CAD build for the part. Positions are in the model's coordinates, mm. Face numbers are marked on the shaded views. A direction names the side the tool comes from. Give positions to 0.01 mm unless a question says otherwise; leave off trailing zeros. Order: outer loops, then holes, each group sorted by start corner. A loop starts at its lowest first (then second) coordinate and runs counter-clockwise, first axis right, second up. Notation, with made-up numbers: M 41,-14 L 60,-14 A35 ccw 60,24 Z; hole C 66.5,87.25 d3. An arc over 180 degrees is marked long. Put each result on its own line as item: value. Start each with the question number.
1) Cut at B-B (y = 13.5). Give the number of separate pieces and of enclosed holes in the cut face, and give its area (3 significant figures).
2) Cut at C-C (z = 2.75). Write the cut outline in (x, y).
3) Pin check, flat tips, straight feed: pin 1 (5 mm diameter, centred on x = 19.5, z = -4, fed in from -Y); pin 2 (3.5 mm diameter, centred on x = -24.5, z = 0, fed in from +Y); pin 3 (1.5 mm diameter, centred on y = 4, z = -3.5, fed in from +X). Stop position of each tip, or through.
4) Cut at A-A (x = -16.5). Write the cut outline in (y, z), and give its area (3 significant figures).
5) Drill centre lines: line 1 (Z direction, x = -19.5, y = 13); line 2 (Y direction, x = 6.5, z = -1); line 3 (X direction, y = 3.5, z = -2.25). Where is each one in solid material? Low to high. Write a range as [from, to].
6) Tool access for the marked faces 1 and 2: list every direction of +Z, -Z, +X, -X, +Y, -Y with a clear straight run to the whole face (end or side of a thin tool).
7) Cut at D-D (x = 8.5). Write the cut outline in (y, z).
```python
from build123d import *

# Parameters (mm, degrees)
SKETCH2_R           = 5
BOSS_EXTRUDE1_DEPTH = 8.44
SKETCH3_R           = 5
BOSS_EXTRUDE2_DEPTH = 6
BOSS_EXTRUDE3_DEPTH = 3
CUT_EXTRUDE1_REACH  = 35.805
SKETCH5_R           = 1.5
SKETCH6_R           = 5
BOSS_EXTRUDE4_DEPTH = 1


with BuildPart() as part:
    # Sketch2 → Boss-Extrude1 (new body)
    with BuildSketch(Plane(origin=(0, 0, 0), x_dir=(1, 0, 0), z_dir=(0, 1, 0))):
        with Locations(Location((0, 0, 0), (0, 0, 270))):
            Circle(SKETCH2_R)
    extrude(amount=BOSS_EXTRUDE1_DEPTH)

    # Sketch3 → Boss-Extrude2 (add)
    with BuildSketch(Plane(origin=(0, 8.44, 0), x_dir=(1, 0, 0), z_dir=(0, 1, 0))):
        with Locations(Location((0, 0, 0), (0, 0, 270))):
            Circle(SKETCH3_R)
    extrude(amount=BOSS_EXTRUDE2_DEPTH)

    # Sketch4 → Boss-Extrude3 (add)
    with BuildSketch(Plane(origin=(0, 14.44, 0), x_dir=(1, 0, 0), z_dir=(0, 1, 0))):
        with BuildLine():
            Line((-0.979591837, -7.939798476), (-25.112244898, -4.962374047))
            ThreePointArc((-25.112244898, -4.962374047), (-29.5, 0), (-25.112244898, 4.962374047))
            Line((-25.112244898, 4.962374047), (-0.979591837, 7.939798476))
            ThreePointArc((-0.979591837, 7.939798476), (0, 8), (0.979591837, 7.939798476))
            Line((0.979591837, 7.939798476), (25.112244898, 4.962374047))
            ThreePointArc((25.112244898, 4.962374047), (29.5, 0), (25.112244898, -4.962374047))
            Line((25.112244898, -4.962374047), (0.979591837, -7.939798476))
            ThreePointArc((0.979591837, -7.939798476), (0, -8), (-0.979591837, -7.939798476))
        make_face()
    extrude(amount=-BOSS_EXTRUDE3_DEPTH)

    # Sketch5 → Cut-Extrude1 (cut, up to next)
    with BuildSketch(Plane(origin=(0, 14.44, 0), x_dir=(1, 0, 0), z_dir=(0, 1, 0)), mode=Mode.PRIVATE) as cut_extrude1_sk1:
        with Locations(Location((24.5, 0, 0), (0, 0, 270))):
            Circle(SKETCH5_R)
    cut_extrude1_tool1 = extrude(cut_extrude1_sk1.sketch, amount=-CUT_EXTRUDE1_REACH, mode=Mode.PRIVATE) & part.part
    # Sketch5 → Cut-Extrude1 (cut, up to next)
    with BuildSketch(Plane(origin=(0, 14.44, 0), x_dir=(1, 0, 0), z_dir=(0, 1, 0)), mode=Mode.PRIVATE) as cut_extrude1_sk2:
        with Locations(Location((20.5, 0, 0), (0, 0, 270))):
            Circle(SKETCH5_R)
    cut_extrude1_tool2 = extrude(cut_extrude1_sk2.sketch, amount=-CUT_EXTRUDE1_REACH, mode=Mode.PRIVATE) & part.part
    # Sketch5 → Cut-Extrude1 (cut, up to next)
    with BuildSketch(Plane(origin=(0, 14.44, 0), x_dir=(1, 0, 0), z_dir=(0, 1, 0)), mode=Mode.PRIVATE) as cut_extrude1_sk3:
        with Locations(Location((16.5, 0, 0), (0, 0, 270))):
            Circle(SKETCH5_R)
    cut_extrude1_tool3 = extrude(cut_extrude1_sk3.sketch, amount=-CUT_EXTRUDE1_REACH, mode=Mode.PRIVATE) & part.part
    # Sketch5 → Cut-Extrude1 (cut, up to next)
    with BuildSketch(Plane(origin=(0, 14.44, 0), x_dir=(1, 0, 0), z_dir=(0, 1, 0)), mode=Mode.PRIVATE) as cut_extrude1_sk4:
        with Locations(Location((12.5, 0, 0), (0, 0, 270))):
            Circle(SKETCH5_R)
    cut_extrude1_tool4 = extrude(cut_extrude1_sk4.sketch, amount=-CUT_EXTRUDE1_REACH, mode=Mode.PRIVATE) & part.part
    # Sketch5 → Cut-Extrude1 (cut, up to next)
    with BuildSketch(Plane(origin=(0, 14.44, 0), x_dir=(1, 0, 0), z_dir=(0, 1, 0)), mode=Mode.PRIVATE) as cut_extrude1_sk5:
        with Locations(Location((8.5, 0, 0), (0, 0, 270))):
            Circle(SKETCH5_R)
    cut_extrude1_tool5 = extrude(cut_extrude1_sk5.sketch, amount=-CUT_EXTRUDE1_REACH, mode=Mode.PRIVATE) & part.part
    # Sketch5 → Cut-Extrude1 (cut, up to next)
    with BuildSketch(Plane(origin=(0, 14.44, 0), x_dir=(1, 0, 0), z_dir=(0, 1, 0)), mode=Mode.PRIVATE) as cut_extrude1_sk6:
        with Locations(Location((-24.5, 0, 0), (0, 0, 270))):
            Circle(SKETCH5_R)
    cut_extrude1_tool6 = extrude(cut_extrude1_sk6.sketch, amount=-CUT_EXTRUDE1_REACH, mode=Mode.PRIVATE) & part.part
    # Sketch5 → Cut-Extrude1 (cut, up to next)
    with BuildSketch(Plane(origin=(0, 14.44, 0), x_dir=(1, 0, 0), z_dir=(0, 1, 0)), mode=Mode.PRIVATE) as cut_extrude1_sk7:
        with Locations(Location((-8.5, 0, 0), (0, 0, 270))):
            Circle(SKETCH5_R)
    cut_extrude1_tool7 = extrude(cut_extrude1_sk7.sketch, amount=-CUT_EXTRUDE1_REACH, mode=Mode.PRIVATE) & part.part
    # Sketch5 → Cut-Extrude1 (cut, up to next)
    with BuildSketch(Plane(origin=(0, 14.44, 0), x_dir=(1, 0, 0), z_dir=(0, 1, 0)), mode=Mode.PRIVATE) as cut_extrude1_sk8:
        with Locations(Location((-12.5, 0, 0), (0, 0, 270))):
            Circle(SKETCH5_R)
    cut_extrude1_tool8 = extrude(cut_extrude1_sk8.sketch, amount=-CUT_EXTRUDE1_REACH, mode=Mode.PRIVATE) & part.part
    # Sketch5 → Cut-Extrude1 (cut, up to next)
    with BuildSketch(Plane(origin=(0, 14.44, 0), x_dir=(1, 0, 0), z_dir=(0, 1, 0)), mode=Mode.PRIVATE) as cut_extrude1_sk9:
        with Locations(Location((-16.5, 0, 0), (0, 0, 270))):
            Circle(SKETCH5_R)
    cut_extrude1_tool9 = extrude(cut_extrude1_sk9.sketch, amount=-CUT_EXTRUDE1_REACH, mode=Mode.PRIVATE) & part.part
    # Sketch5 → Cut-Extrude1 (cut, up to next)
    with BuildSketch(Plane(origin=(0, 14.44, 0), x_dir=(1, 0, 0), z_dir=(0, 1, 0)), mode=Mode.PRIVATE) as cut_extrude1_sk10:
        with Locations(Location((-20.5, 0, 0), (0, 0, 270))):
            Circle(SKETCH5_R)
    cut_extrude1_tool10 = extrude(cut_extrude1_sk10.sketch, amount=-CUT_EXTRUDE1_REACH, mode=Mode.PRIVATE) & part.part
    add(cut_extrude1_tool1.solids().sort_by_distance((24.5, 14.44, 0))[0], mode=Mode.SUBTRACT)
    add(cut_extrude1_tool2.solids().sort_by_distance((20.5, 14.44, 0))[0], mode=Mode.SUBTRACT)
    add(cut_extrude1_tool3.solids().sort_by_distance((16.5, 14.44, 0))[0], mode=Mode.SUBTRACT)
    add(cut_extrude1_tool4.solids().sort_by_distance((12.5, 14.44, 0))[0], mode=Mode.SUBTRACT)
    add(cut_extrude1_tool5.solids().sort_by_distance((8.5, 14.44, 0))[0], mode=Mode.SUBTRACT)
    add(cut_extrude1_tool6.solids().sort_by_distance((-24.5, 14.44, 0))[0], mode=Mode.SUBTRACT)
    add(cut_extrude1_tool7.solids().sort_by_distance((-8.5, 14.44, 0))[0], mode=Mode.SUBTRACT)
    add(cut_extrude1_tool8.solids().sort_by_distance((-12.5, 14.44, 0))[0], mode=Mode.SUBTRACT)
    add(cut_extrude1_tool9.solids().sort_by_distance((-16.5, 14.44, 0))[0], mode=Mode.SUBTRACT)
    add(cut_extrude1_tool10.solids().sort_by_distance((-20.5, 14.44, 0))[0], mode=Mode.SUBTRACT)

    # Sketch6 → Boss-Extrude4 (add)
    with BuildSketch(Plane(origin=(0, 14.44, 0), x_dir=(1, 0, 0), z_dir=(0, 1, 0))):
        with Locations(Location((0, 0, 0), (0, 0, 270))):
            Circle(SKETCH6_R)
    extrude(amount=BOSS_EXTRUDE4_DEPTH)


solid = part.part
```
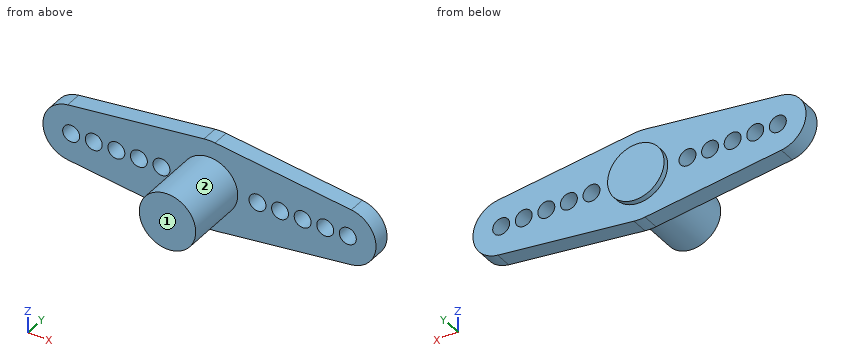
Solution:
1. separate pieces: 1
1. enclosed holes: 10
1. area: 650 mm²
2. outline: M -28.68,11.44 L -4.18,11.44 L -4.18,0 L 4.18,0 L 4.18,11.44 L 28.68,11.44 L 28.68,14.44 L 4.18,14.44 L 4.18,15.44 L -4.18,15.44 L -4.18,14.44 L -28.68,14.44 Z
3. pin 1: y = 11.44
3. pin 2: y = 14.44
3. pin 3: x = 4.18
4. outline: M 11.44,-6.02 L 14.44,-6.02 L 14.44,-1.5 L 11.44,-1.5 Z; M 11.44,1.5 L 14.44,1.5 L 14.44,6.02 L 11.44,6.02 Z
4. area: 27.1 mm²
5. line 1: [-5.65, -1.12], [1.12, 5.65]
5. line 2: [11.44, 14.44]
5. line 3: [-4.47, 4.47]
6. face 1: +Z, -Z, +X, -X, -Y
6. face 2: -Y
7. outline: M 11.44,-7.01 L 14.44,-7.01 L 14.44,-1.5 L 11.44,-1.5 Z; M 11.44,1.5 L 14.44,1.5 L 14.44,7.01 L 11.44,7.01 Z
